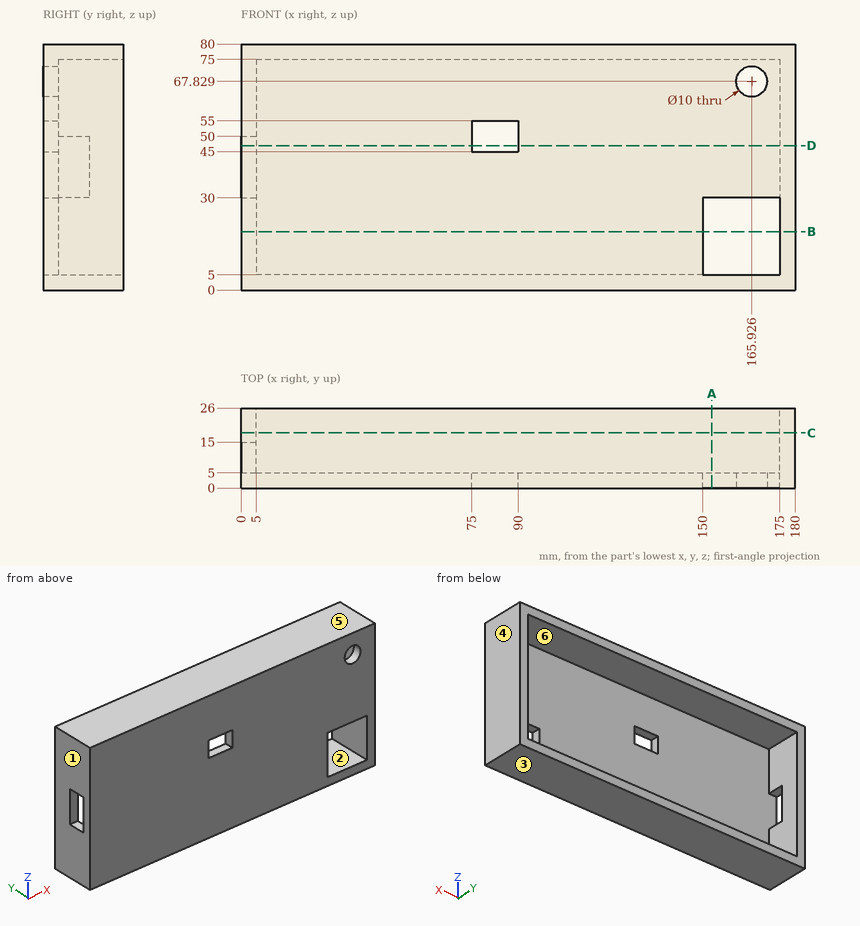
Design review of the part shown in the three views and the two pictorial views. Dimensions are in mm from the part's minimum x, y and z. A direction names the side the tool comes from. Give positions to 0.01 mm unless a question says otherwise; leave off trailing zeros. Write each loop counter-clockwise with the first axis right and the second up, starting at its lowest first coordinate (ties: lowest second). Pieces come first, ordered by that corner, then holes.
(1) Wall thickness on line 1 along Z through (x, y) = (49, 14); line 2 along X through (y, z) = (17.75, 11.5); line 3 along Z through (x, y) = (81.5, 1.75): over which ranges is each line inside the solid? List them lowest first.
Checked values:
line 1: z = 0 to 5, 75 to 80
line 2: x = 0 to 5, 175 to 180
line 3: z = 0 to 45, 55 to 80
(2) Tool access review of the marked faces 5 and 6: name each direction out of +Z, -Z, +X, -X, +Y, -Y from which nothing blocks a thin tool from reaching the whole face with its end or side.
Checked values:
face 5: +Z, +X, -X, +Y, -Y
face 6: +Y
(3) Mouldability with a two-part tool opening along X and no side actions: class the marked faces 1, 2, 3 and 4 as +X half, -X half, draft (parallel to the pull), parting line (faces both ways), or undercut.
Checked values:
face 1: -X half
face 2: undercut
face 3: draft
face 4: +X half
(4) Add section B-B (z = 19). Give the boundary of the cut face in (x, y), and give its area (3 significant figures).
Checked values:
outline: (0, 0) - (150, 0) - (150, 5) - (5, 5) - (5, 26) - (0, 26) - close; (175, 0) - (180, 0) - (180, 26) - (175, 26) - close
area: 985 mm2
(5) Add section D-D (z = 47). Give the boundary of the cut face in (x, y).
Checked values:
outline: (0, 0) - (75, 0) - (75, 5) - (0, 5) - close; (0, 15) - (5, 15) - (5, 26) - (0, 26) - close; (90, 0) - (180, 0) - (180, 26) - (175, 26) - (175, 5) - (90, 5) - close
(6) Clearance check with flat-ended pins moving along their axes: pin 1 Ø10 at (x, y) = (82.5, 5) entering from -Z; pin 2 Ø21 at (x, z) = (97.5, 38) entering from +Y. State where each tip first meets the part, or that it passes through.
Checked values:
pin 1: stops at z = 0
pin 2: stops at y = 5
(7) Add section C-C (y = 18). Give the boundary of the cut face in (x, z), and give its area (3 significant figures).
Checked values:
outline: (0, 0) - (180, 0) - (180, 80) - (0, 80) - close; hole (5, 5) - (175, 5) - (175, 75) - (5, 75) - close
area: 2,500 mm2
(8) Add section A-A (x = 153). Give the boundary of the cut face in (y, z).
Checked values:
outline: (0, 0) - (26, 0) - (26, 5) - (0, 5) - close; (0, 30) - (5, 30) - (5, 75) - (26, 75) - (26, 80) - (0, 80) - close
